The listing builds one solid part. Answer for the finished solid, in the listing's coordinates (mm). Coordinates: 2 decimals unless noted, no trailing zeros. Order: outer loops, then holes, each group sorted by start corner. A loop starts at its lowest first (then second) coordinate and runs counter-clockwise, first axis right, second up. Notation, with made-up numbers: (14.25, 15) -> (41.25, 15) arc R14 cw to (41.25, 33) -> close; hole circle Ø7 at (81.5, 29). An arc over 180 degrees is marked (long way). Answer in a Markdown table with one row per item.
```python
from build123d import *

# Parameters (mm, degrees)
EXTRUDE_500_DEPTH = 6


with BuildPart() as part:
    # Sketch 492 → Extrude 500 (new body)
    with BuildSketch(Plane(origin=(0, 0, 0), x_dir=(0, 0, -1), z_dir=(1, 0, 0))):
        Polygon((-593.846153846, -224.461538462), (6.153846154, -224.461538462), (6.153846154, -164.461538462), (-233.846153846, 335.538461538), (-293.846153846, 335.538461538), (-293.846153846, -164.461538462), (-593.846153846, -164.461538462), align=None)
        Polygon((-233.846153846, -164.461538462), (-60.400192041, -164.461538462), (-233.846153846, 196.8842153), align=None, mode=Mode.SUBTRACT)
    extrude(amount=EXTRUDE_500_DEPTH)


solid = part.part
```
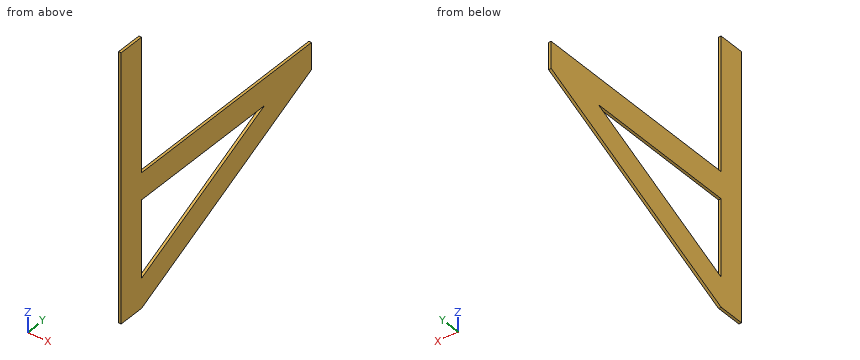
(1) A cutting plane is placed at B-B, the plane y = 3.5. Determine the outline of the cut face in (x, z), then the cut area to 3 significant figures.
Check values:
| item | result |
|---|---|
| outline | (0, 74.47) -> (6, 74.47) -> (6, 141.02) -> (0, 141.02) -> close; (0, 233.85) -> (6, 233.85) -> (6, 293.85) -> (0, 293.85) -> close |
| area | 759 mm² |
(2) A cutting plane is placed at C-C, the plane z = 470.5. Determine the outline of the cut face in (x, y), then the cut area to 3 significant figures.
Check values:
| item | result |
|---|---|
| outline | (0, -224.46) -> (6, -224.46) -> (6, -164.46) -> (0, -164.46) -> close |
| area | 360 mm² |
(3) Flat-ended cylindrical pins translate along their axes: pin 1 (2 mm diameter, centred on x = 0.5, y = -30.5, fed in from -Z); pin 2 (2 mm diameter, centred on x = 4.5, y = 121, fed in from -Z); pin 3 (3 mm diameter, centred on x = 2.5, y = 56.5, fed in from +Z). Find the tip coordinate at first contact, or state that the pin passes through.
Check values:
| item | result |
|---|---|
| pin 1 | z = 57.67 |
| pin 2 | z = 130.39 |
| pin 3 | z = 293.85 |
(4) Find the intervals of material crossed by line 1 along Y through (x, z) = (4.15, 364); line 2 along Y through (x, z) = (5.6, 160.5); line 3 along Z through (x, y) = (4.05, -60), in increasing order. Write a range as from..to.
Check values:
| item | result |
|---|---|
| line 1 | -224.46..-164.46 |
| line 2 | -224.46..-164.46, 44.08..182.73 |
| line 3 | 43.99..110.54, 233.85..293.85 |
(5) A cutting plane is placed at D-D, the plane y = 287. Determine the outline of the cut face in (x, z), then the cut area to 3 significant figures.
Check values:
| item | result |
|---|---|
| outline | (0, 210.55) -> (6, 210.55) -> (6, 293.85) -> (0, 293.85) -> close |
| area | 500 mm² |
(6) A cutting plane is placed at A-A, the plane x = 4.45. Determine the outline of the cut face in (y, z), then the cut area to 3 significant figures.
Check values:
| item | result |
|---|---|
| outline | (-224.46, -6.15) -> (-164.46, -6.15) -> (335.54, 233.85) -> (335.54, 293.85) -> (-164.46, 293.85) -> (-164.46, 593.85) -> (-224.46, 593.85) -> close; hole (-164.46, 60.4) -> (196.88, 233.85) -> (-164.46, 233.85) -> close |
| area | 94,700 mm² |
